from build123d import *

# Parameters (mm, degrees)
F0_W      = 4
F0_H      = 17
F1_DEPTH  = 1.8
F3_DEPTH  = 22
F4_W      = 44
F4_H      = 59.4
F5_DEPTH  = 6
F6_W      = 2.25
F6_H      = 20
F7_DEPTH  = 10
F9_DEPTH  = 20
F11_DEPTH = 17
F13_DEPTH = 20
F15_DEPTH = 17
F17_DEPTH = 45
F18_R     = 3.375
F19_DEPTH = 3
F20_R     = 1.05
F21_DEPTH = 7.5
F22_W     = 10
F22_H     = 2
F23_DEPTH = 2.5
F25_START = 1
F24_W     = 2.95
F24_H     = 2.1
F25_DEPTH = 15
F26_W     = 5
F26_H     = 5
F26_R     = 1.2
F26_W_2   = 6
F26_H_2   = 6
F27_DEPTH = 4


# Not quite as in the source:
# - a feature names something its author has since deleted; it is built from what else it names


with BuildPart() as f1:
    # F0 (on Top) → F1 (new body)
    with BuildSketch(Plane.XY):
        Polygon((-12.630645159, 54.2783500865), (-56.630645159, 54.2783500865), (-56.630645159, 33.0783500865), (-54.380645159, 33.0783500865), (-54.380645159, 16.0783500865), (-56.630645159, 16.0783500865), (-56.630645159, -5.1216499135), (-12.630645159, -5.1216499135), (-12.630645159, 16.0783500865), (-14.880645159, 16.0783500865), (-14.880645159, 33.0783500865), (-12.630645159, 33.0783500865), align=None)
        with Locations((-18.730645159, 4.8783500865)):
            Rectangle(F0_W, F0_H, mode=Mode.SUBTRACT)
    extrude(amount=F1_DEPTH)

    # F2 (on face) → F3 (join)
    with BuildSketch(Plane.XY.offset(1.8)):
        Polygon((-12.630645159, 33.0783500865), (-12.630645159, 54.2783500865), (-56.630645159, 54.2783500865), (-56.630645159, 33.0783500865), (-54.380645159, 33.0783500865), (-54.380645159, 16.0783500865), (-56.630645159, 16.0783500865), (-56.630645159, -5.1216499135), (-12.630645159, -5.1216499135), (-12.630645159, 16.0783500865), (-14.880645159, 16.0783500865), (-14.880645159, 33.0783500865), align=None)
        Polygon((-55.130645159, 34.5783500865), (-55.130645159, 52.7783500865), (-14.130645159, 52.7783500865), (-14.130645159, 34.5783500865), (-16.380645159, 34.5783500865), (-16.380645159, 14.5783500865), (-14.130645159, 14.5783500865), (-14.130645159, -3.6216499135), (-16.730645159, -3.6216499135), (-20.730645159, -3.6216499135), (-55.130645159, -3.6216499135), (-55.130645159, 14.5783500865), (-52.880645159, 14.5783500865), (-52.880645159, 34.5783500865), align=None, mode=Mode.SUBTRACT)
    extrude(amount=F3_DEPTH)

    # F4 (on face) → F5 (join)
    with BuildSketch(Plane.XY.offset(23.8)):
        with Locations((-34.630645159, 24.5783500865)):
            Rectangle(F4_W, F4_H)
        Polygon((-55.130645159, 34.5783500865), (-55.130645159, 52.7783500865), (-14.130645159, 52.7783500865), (-14.130645159, 34.5783500865), (-16.380645159, 34.5783500865), (-16.380645159, 14.5783500865), (-14.130645159, 14.5783500865), (-14.130645159, -3.6216499135), (-55.130645159, -3.6216499135), (-55.130645159, 14.5783500865), (-52.880645159, 14.5783500865), (-52.880645159, 34.5783500865), align=None, mode=Mode.SUBTRACT)
    extrude(amount=F5_DEPTH)

    # F6 (on face) → F7 (cut)
    with BuildSketch(Plane.XY.offset(29.8)):
        with Locations((-54.005645159, 24.5783500865)):
            Rectangle(F6_W, F6_H)
        with Locations((-15.255645159, 24.5783500865)):
            Rectangle(F6_W, F6_H)
    extrude(amount=-F7_DEPTH, mode=Mode.SUBTRACT)

    # F8 (on face) → F9 (cut)
    with BuildSketch(Plane.XZ.offset(-14.5783500865)):
        Polygon((-52.880645159, 19.8), (-55.130645159, 19.8), (-52.880645159, 17.55), align=None)
    extrude(amount=-F9_DEPTH, mode=Mode.SUBTRACT)

    # F10 (on face) → F11 (cut)
    with BuildSketch(Plane.XZ.offset(-33.0783500865)):
        Polygon((-56.630645159, 24.8), (-56.630645159, 23.8), (-55.880645159, 23.8), (-54.380645159, 23.8), align=None)
    extrude(amount=F11_DEPTH, mode=Mode.SUBTRACT)

    # F12 (on face) → F13 (cut)
    with BuildSketch(Plane(origin=(0, 34.5783500865, 0), x_dir=(-1, 0, 0), z_dir=(0, 1, 0))):
        Polygon((16.380645159, 17.55), (16.380645159, 19.8), (14.130645159, 19.8), align=None)
    extrude(amount=-F13_DEPTH, mode=Mode.SUBTRACT)

    # F14 (on face) → F15 (cut)
    with BuildSketch(Plane(origin=(0, 16.0783500865, 0), x_dir=(-1, 0, 0), z_dir=(0, 1, 0))):
        Polygon((12.630645159, 24.8), (12.630645159, 23.8), (14.880645159, 23.8), align=None)
    extrude(amount=F15_DEPTH, mode=Mode.SUBTRACT)

    # F16 (on face) → F17 (cut)
    with BuildSketch(Plane.YZ.offset(-12.630645159)):
        Polygon((32.2783500865, 29.8), (-5.1216499135, 29.8), (-5.1216499135, 17.8), align=None)
    extrude(amount=-F17_DEPTH, mode=Mode.SUBTRACT)

    # F18 (on face) → F19 (cut)
    with BuildSketch(Plane(origin=(0, 54.2783500865, 0), x_dir=(-1, 0, 0), z_dir=(0, 1, 0))):
        with Locations((34.630645159, 24.8)):
            Circle(F18_R)
    extrude(amount=-F19_DEPTH, mode=Mode.SUBTRACT)

    # F20 (on face) → F21 (join)
    with BuildSketch(Plane.XY.offset(29.8)):
        with BuildLine():
            Line((-55.130645159, 52.7783500865), (-55.130645159, 48.7783500865))
            ThreePointArc((-55.130645159, 48.7783500865), (-52.3091414621, 49.9568463896), (-51.130645159, 52.7783500865))
            Line((-51.130645159, 52.7783500865), (-55.130645159, 52.7783500865))
        make_face()
        with Locations((-53.6807930499, 51.4078039413)):
            Circle(F20_R, mode=Mode.SUBTRACT)
        with BuildLine():
            Line((-14.130645159, 52.7783500865), (-18.130645159, 52.7783500865))
            ThreePointArc((-18.130645159, 52.7783500865), (-16.952148856, 49.9568463896), (-14.130645159, 48.7783500865))
            Line((-14.130645159, 48.7783500865), (-14.130645159, 52.7783500865))
        make_face()
        with Locations((-15.5804972681, 51.4078039413)):
            Circle(F20_R, mode=Mode.SUBTRACT)
    extrude(amount=-F21_DEPTH)

    # F22 (on face) → F23 (cut)
    with BuildSketch(Plane.XZ.offset(5.1216499135)):
        with Locations((-34.630645159, 14.8)):
            Rectangle(F22_W, F22_H)
    extrude(amount=-F23_DEPTH, mode=Mode.SUBTRACT)

    # F24 (on face) → F25 (join)
    with BuildSketch(Plane.XZ.offset(-33.0783500865).offset(F25_START)):
        with Locations((-11.155645159, 17.575)):
            Rectangle(F24_W, F24_H)
        with BuildLine():
            Line((-14.880645159, 9.525), (-14.880645159, 6))
            ThreePointArc((-14.880645159, 6), (-13.2978940887, 8.5959050075), (-12.630645159, 11.5621488653))
            Line((-12.630645159, 11.5621488653), (-12.630645159, 14.525))
            Line((-12.630645159, 14.525), (-12.630645159, 16.525))
            Line((-12.630645159, 16.525), (-12.630645159, 18.625))
            Line((-12.630645159, 18.625), (-13.680645159, 18.625))
            Line((-13.680645159, 18.625), (-14.880645159, 9.525))
        make_face()
        Polygon((-12.630645159, 14.525), (-12.630645159, 11.5621488653), (-11.630645159, 14.525), align=None)
        with BuildLine():
            Line((-57.630645159, 14.525), (-56.630645159, 11.5621488653))
            ThreePointArc((-56.630645159, 11.5621488653), (-55.9633962294, 8.5959050075), (-54.380645159, 6))
            Line((-54.380645159, 6), (-54.380645159, 8.2336284751))
            Line((-54.380645159, 8.2336284751), (-55.0399858184, 19.425))
            Line((-55.0399858184, 19.425), (-59.580645159, 19.425))
            Line((-59.580645159, 19.425), (-59.580645159, 17.325))
            Line((-59.580645159, 17.325), (-57.0257989239, 16.632160343))
            Line((-57.0257989239, 16.632160343), (-56.630645159, 15.525))
            Line((-56.630645159, 15.525), (-56.630645159, 14.525))
            Line((-56.630645159, 14.525), (-57.630645159, 14.525))
        make_face()
    extrude(amount=F25_DEPTH)

    # F26 (on face) → F27 (join)
    with BuildSketch(Plane.XY.offset(1.8)):
        with Locations((-48.730645159, 14.2783500865)):
            Rectangle(F26_W, F26_H)
        with Locations((-48.730645159, 14.2783500865)):
            Circle(F26_R, mode=Mode.SUBTRACT)
        with Locations((-26.330645159, 0.0783500865)):
            Rectangle(F26_W, F26_H)
        with Locations((-26.330645159, 0.0783500865)):
            Circle(F26_R, mode=Mode.SUBTRACT)
        with Locations((-17.130645159, 45.7783500865)):
            Rectangle(F26_W_2, F26_H_2)
        with Locations((-17.130645159, 45.7783500865)):
            Circle(F26_R, mode=Mode.SUBTRACT)
        with Locations((-37.6969575882, 45.7783500865)):
            Rectangle(F26_W_2, F26_H_2)
    extrude(amount=F27_DEPTH)


solid = f1.part
Geometry check sheet. Reference: the model listing, model coordinates, mm. A direction names the side the tool comes from. Give positions to 0.01 mm unless a question says otherwise; leave off trailing zeros. Loops run counter-clockwise (first coordinate to the right, second up) from the corner with the lowest first, then second, coordinate; pieces in that order, holes last. Notation, with made-up numbers: (21.5, 19.5) -> (58.5, 19.5) arc R25 ccw to (58.5, 41.5) -> close; hole circle Ø9 at (41.5, 5). An arc over 180 degrees is marked (long way). Answer in a Markdown table with one row per item. Add a question column.
1) Material ranges on probe 1 along Y at (x, z) = (-54, 15); probe 2 along Y at (x, z) = (-23.5, 5.5); probe 3 along X at (y, z) = (8, 19.5), recorded low to high. Write a range as from..to.
2) Gauge pin test, flat ends, axial feed: P1, Ø2.5, axis at x = -26, y = 0, coming from the +Z side; P2, Ø2, axis at y = 1, z = 0.5, coming from the -X side; P3, Ø2, axis at y = 31, z = 5.5, coming from the +X side; P4, Ø1, axis at y = 23, z = 20, coming from the -X side. Record the tip position at first contact, or that the pin passes through.
3) Cross-section at A-A on x = -19. Record the boundary of the cut face in (y, z).
4) Set-up check for faces 4 (the face through (-56, 32.078, 14)), 5 (the face through (-51.231, 14, 4)), 6 (the face through (-35, 52.778, 16)), 7 (the face through (-14, 16.078, 12)): record each of +Z, -Z, +X, -X, +Y, -Y from which the full face is reachable in a straight line by a thin tool's end or side.
5) Cross-section at B-B on y = 36. Record the boundary of the cut face in (x, z), and give its area (3 significant figures).
6) Draft check along Y on faces 1 (the face through (-52.34, 49.926, 26.102)), 2 (the face through (-56.631, 5, 9)), 3 (the face through (-57, 25, 19.425)). Enter one of: pulls with the +Y half, pulls with the -Y half, needs draft (parallel to the pull), parting line crosses it, or undercut.
7) Cross-section at C-C on y = 18. State how many separate pieces and enclosed holes the cut face has, and give its area (3 significant figures).
Outcome:
| question | item | result |
|---|---|---|
| 1 | probe 1 | y = -5.12..-3.62, 14.58..34.58, 52.78..54.28 |
| 1 | probe 2 | y = -5.12..-3.62, 52.78..54.28 |
| 1 | probe 3 | x = -56.63..-55.13, -14.13..-12.63 |
| 2 | P1 | stops at z = 5.8 |
| 2 | P2 | stops at x = -56.63 |
| 2 | P3 | stops at x = -14.48 |
| 2 | P4 | passes through |
| 3 | outline | (-5.12, 0) -> (-3.62, 0) -> (-3.62, 18.28) -> (-5.12, 17.8) -> close; (13.38, 0) -> (54.28, 0) -> (54.28, 29.8) -> (52.78, 29.8) -> (52.78, 1.8) -> (48.78, 1.8) -> (48.78, 5.8) -> (42.78, 5.8) -> (42.78, 1.8) -> (13.38, 1.8) -> close |
| 4 | face 4 | -Z, -X |
| 4 | face 5 | +Z |
| 4 | face 6 | none |
| 4 | face 7 | -Z, +X |
| 5 | outline | (-56.63, 0) -> (-12.63, 0) -> (-12.63, 29.8) -> (-14.13, 29.8) -> (-14.13, 1.8) -> (-55.13, 1.8) -> (-55.13, 29.8) -> (-56.63, 29.8) -> close |
| 5 | area | 163 mm^2 |
| 6 | face 1 | pulls with the -Y half |
| 6 | face 2 | needs draft |
| 6 | face 3 | undercut |
| 7 | separate pieces | 3 |
| 7 | enclosed holes | 0 |
| 7 | area | 181 mm^2 |
